from build123d import *

# Parameters (mm, degrees)
SZKIC1_W                                            = 750
SZKIC1_H                                            = 500
WYCI_GNI_CIE1_DEPTH                                 = 80
SFAZOWANIE1_SIZE                                    = 10
WYCI_GNI_CIE2_REACH                                 = 459.739
SZKIC2_R                                            = 52.5
WYCI_GNI_CIE3_REACH                                 = 459.739
SZKIC3_R                                            = 37
SFAZOWANIE2_SIZE                                    = 2
WYTNIJ_WYCI_GNI_CIE1_DEPTH                          = 0.1
SZKIC5_R                                            = 50
WYTNIJ_WYCI_GNI_CIE3_DEPTH                          = 20
POG_BIENIE_WALCOWE_POD_M8_WKR_T_Z_BEM_W_D           = 9
POG_BIENIE_WALCOWE_POD_M8_WKR_T_Z_BEM_W_CBORE_D     = 15
POG_BIENIE_WALCOWE_POD_M8_WKR_T_Z_BEM_W_CBORE_DEPTH = 8.6
OTW_R_POD_RUB_M201_D                                = 22


with BuildPart() as part:
    # Szkic1 → Wyciągnięcie1 (new body)
    with BuildSketch(Plane(origin=(0, 0, 0), x_dir=(1, 0, 0), z_dir=(0, 1, 0))):
        Rectangle(SZKIC1_W, SZKIC1_H)
    extrude(amount=WYCI_GNI_CIE1_DEPTH)

    # Sfazowanie1
    sfazowanie1_edges = [part.edges().sort_by_distance(p)[0] for p in [
        (375, 40, 250),
        (-375, 40, 250),
        (-375, 40, -250),
        (375, 40, -250),
    ]]
    chamfer(sfazowanie1_edges, length=SFAZOWANIE1_SIZE)

    # Szkic2 → Wyciągnięcie2 (cut, up to next)
    with BuildSketch(Plane(origin=(0, 80, 0), x_dir=(1, 0, 0), z_dir=(0, 1, 0)), mode=Mode.PRIVATE) as wyci_gni_cie2_sk1:
        with Locations(Location((-300, 175, 0), (0, 0, 270))):
            Circle(SZKIC2_R)
    wyci_gni_cie2_tool1 = extrude(wyci_gni_cie2_sk1.sketch, amount=-WYCI_GNI_CIE2_REACH, mode=Mode.PRIVATE) & part.part
    # Szkic2 → Wyciągnięcie2 (cut, up to next)
    with BuildSketch(Plane(origin=(0, 80, 0), x_dir=(1, 0, 0), z_dir=(0, 1, 0)), mode=Mode.PRIVATE) as wyci_gni_cie2_sk2:
        with Locations(Location((300, 175, 0), (0, 0, 90))):
            Circle(SZKIC2_R)
    wyci_gni_cie2_tool2 = extrude(wyci_gni_cie2_sk2.sketch, amount=-WYCI_GNI_CIE2_REACH, mode=Mode.PRIVATE) & part.part
    # Szkic2 → Wyciągnięcie2 (cut, up to next)
    with BuildSketch(Plane(origin=(0, 80, 0), x_dir=(1, 0, 0), z_dir=(0, 1, 0)), mode=Mode.PRIVATE) as wyci_gni_cie2_sk3:
        with Locations(Location((-300, -175, 0), (0, 0, 90))):
            Circle(SZKIC2_R)
    wyci_gni_cie2_tool3 = extrude(wyci_gni_cie2_sk3.sketch, amount=-WYCI_GNI_CIE2_REACH, mode=Mode.PRIVATE) & part.part
    # Szkic2 → Wyciągnięcie2 (cut, up to next)
    with BuildSketch(Plane(origin=(0, 80, 0), x_dir=(1, 0, 0), z_dir=(0, 1, 0)), mode=Mode.PRIVATE) as wyci_gni_cie2_sk4:
        with Locations(Location((300, -175, 0), (0, 0, 270))):
            Circle(SZKIC2_R)
    wyci_gni_cie2_tool4 = extrude(wyci_gni_cie2_sk4.sketch, amount=-WYCI_GNI_CIE2_REACH, mode=Mode.PRIVATE) & part.part
    add(wyci_gni_cie2_tool1.solids().sort_by_distance((-300, 80, -175))[0], mode=Mode.SUBTRACT)
    add(wyci_gni_cie2_tool2.solids().sort_by_distance((300, 80, -175))[0], mode=Mode.SUBTRACT)
    add(wyci_gni_cie2_tool3.solids().sort_by_distance((-300, 80, 175))[0], mode=Mode.SUBTRACT)
    add(wyci_gni_cie2_tool4.solids().sort_by_distance((300, 80, 175))[0], mode=Mode.SUBTRACT)

    # Szkic3 → Wyciągnięcie3 (cut, up to next)
    with BuildSketch(Plane(origin=(0, 80, 0), x_dir=(1, 0, 0), z_dir=(0, 1, 0)), mode=Mode.PRIVATE) as wyci_gni_cie3_sk1:
        with Locations(Location((-250, 0, 0), (0, 0, 270))):
            Circle(SZKIC3_R)
    wyci_gni_cie3_tool1 = extrude(wyci_gni_cie3_sk1.sketch, amount=-WYCI_GNI_CIE3_REACH, mode=Mode.PRIVATE) & part.part
    # Szkic3 → Wyciągnięcie3 (cut, up to next)
    with BuildSketch(Plane(origin=(0, 80, 0), x_dir=(1, 0, 0), z_dir=(0, 1, 0)), mode=Mode.PRIVATE) as wyci_gni_cie3_sk2:
        with Locations(Location((250, 0, 0), (0, 0, 90))):
            Circle(SZKIC3_R)
    wyci_gni_cie3_tool2 = extrude(wyci_gni_cie3_sk2.sketch, amount=-WYCI_GNI_CIE3_REACH, mode=Mode.PRIVATE) & part.part
    add(wyci_gni_cie3_tool1.solids().sort_by_distance((-250, 80, 0))[0], mode=Mode.SUBTRACT)
    add(wyci_gni_cie3_tool2.solids().sort_by_distance((250, 80, 0))[0], mode=Mode.SUBTRACT)

    # Sfazowanie2
    sfazowanie2_edges = [part.edges().sort_by_distance(p)[0] for p in [
        (375, 0, 0),
        (375, 80, 0),
        (0, 0, 250),
        (-375, 0, 0),
        (0, 0, -250),
        (-370, 0, 245),
        (-370, 0, -245),
        (370, 0, -245),
        (370, 0, 245),
        (0, 80, 250),
        (0, 80, -250),
        (-375, 80, 0),
        (-370, 80, 245),
        (-370, 80, -245),
        (370, 80, -245),
        (370, 80, 245),
        (-300, 0, -227.5),
        (-300, 80, -227.5),
        (300, 0, -122.5),
        (300, 80, -122.5),
        (-300, 0, 227.5),
        (-300, 80, 227.5),
        (300, 0, 122.5),
        (300, 80, 122.5),
        (-250, 0, -37),
        (-250, 80, -37),
        (250, 0, 37),
        (250, 80, 37),
    ]]
    chamfer(sfazowanie2_edges, length=SFAZOWANIE2_SIZE)

    # Szkic4 → Wytnij-wyciągnięcie1 (cut)
    with BuildSketch(Plane(origin=(0, 0, -250), x_dir=(-1, 0, 0), z_dir=(0, 0, -1))):
        Polygon((-363.299129796, 74.48655724), (-362.394621346, 76.295574139), (-361.625789164, 76.295574139), (-361.625789164, 72.270511538), (-362.394621346, 72.270511538), (-362.394621346, 74.283042838), align=None)
        Polygon((-358.2791079, 76.295574139), (-359.952448532, 73.808175902), (-358.2791079, 73.808175902), (-358.2791079, 72.270511538), (-357.666731233, 72.270511538), (-357.666731233, 76.295574139), align=None)
    extrude(amount=-WYTNIJ_WYCI_GNI_CIE1_DEPTH, mode=Mode.SUBTRACT)

    # Szkic5 → Wytnij-wyciągnięcie3 (cut)
    with BuildSketch(Plane(origin=(0, 80, 0), x_dir=(-1, 0, 0), z_dir=(0, -1, 0))):
        with Locations(Location((0, 0, 0), (0, 0, 90))):
            Circle(SZKIC5_R)
    extrude(amount=WYTNIJ_WYCI_GNI_CIE3_DEPTH, mode=Mode.SUBTRACT)

    # Pogłębienie walcowe pod M8 Wkręt z łbem walcowym z gniazdem sześciokątnym1 (through all)
    with Locations(Plane(origin=(-68.13672833, 0, 0), x_dir=(0, 0, -1), z_dir=(0, -1, 0))):
        with Locations((0, 0), (-59.008137665, 34.068364165), (-59.008137665, 102.205092495), (0, 136.27345666), (59.008137665, 102.205092495), (59.008137665, 34.068364165)):
            CounterBoreHole(POG_BIENIE_WALCOWE_POD_M8_WKR_T_Z_BEM_W_D / 2, POG_BIENIE_WALCOWE_POD_M8_WKR_T_Z_BEM_W_CBORE_D / 2, POG_BIENIE_WALCOWE_POD_M8_WKR_T_Z_BEM_W_CBORE_DEPTH)

    # Otwór pod śrubę M201 (through all)
    with Locations(Plane(origin=(0, 0, 0), x_dir=(-1, 0, 0), z_dir=(0, -1, 0))):
        with Locations((0, 0)):
            Hole(OTW_R_POD_RUB_M201_D / 2)


solid = part.part
Source: CAD feature listing. Evaluate the final solid. Frame: model axes, mm. A direction names the side the tool comes from. Round coordinates to 2 decimals unless told otherwise and drop trailing zeros. Order: outer loops, then holes, each group sorted by start corner. A loop starts at its lowest first (then second) coordinate and runs counter-clockwise, first axis right, second up. Notation, with made-up numbers: (-10.75, 23.25) - (7.25, 23.25) arc R5 cw to (7.25, 29.25) - close; hole circle Ø2 at (61.5, 88). An arc over 180 degrees is marked (long way). Use a Markdown table: item, result. Add a question column.
1. Line query: probe 1 along X at (y, z) = (60, 175); probe 2 along X at (y, z) = (62, 0); probe 3 along Z at (x, y) = (-296, 61.5). Output: solid intervals per line, ascending.
2. Section query C-C (y = 35). Give the number of separate pieces and of enclosed holes in the cut face, then the cut area to 3 significant figures.
3. Section query A-A (x = 300). Return the cut outline in (y, z), then the cut area to 3 significant figures.
4. Section query B-B (x = 0). Return the cut outline in (y, z), then the cut area to 3 significant figures.
5. Set-up query: faces 5 (the cylindrical face through (247.947, 40.532, -168.166)), 6 (the flat face through (12, 60, 1)), 7 (the flat face through (63, 8.6, 0)). Return all of +Z, -Z, +X, -X, +Y, -Y with unobstructed straight access to the full face (end or side cutting, diameter ignored); none if empty.
6. Mould query, pull axis X, two halves, no side actions, for faces 1 (the flat face through (-5, 39, 250)), 2 (the cylindrical face through (-40.722, 4.24, 55.547)), 3 (the flat face through (375, 39, 3)), 4 (the flat face through (-375, 39, 3)). Classes: +X half, -X half, draft (parallel to the pull), parting line (faces both ways), or undercut.
Derived:
| question | item | result |
|---|---|---|
| 1 | probe 1 | -375 to -352.5, -247.5 to 247.5, 352.5 to 375 |
| 1 | probe 2 | -375 to -287, -213 to -72.64, -63.64 to -50, 50 to 63.64, 72.64 to 213, 287 to 375 |
| 1 | probe 3 | -250 to -227.35, -122.65 to 122.65, 227.35 to 250 |
| 2 | separate pieces | 1 |
| 2 | enclosed holes | 13 |
| 2 | area | 331,000 mm2 |
| 3 | outline | (0, -248) - (2, -250) - (78, -250) - (80, -248) - (80, -229.5) - (78, -227.5) - (2, -227.5) - (0, -229.5) - close; (0, -120.5) - (2, -122.5) - (78, -122.5) - (80, -120.5) - (80, 120.5) - (78, 122.5) - (2, 122.5) - (0, 120.5) - close; (0, 229.5) - (2, 227.5) - (78, 227.5) - (80, 229.5) - (80, 248) - (78, 250) - (2, 250) - (0, 248) - close |
| 3 | area | 23,200 mm2 |
| 4 | outline | (0, -248) - (2, -250) - (78, -250) - (80, -248) - (80, -50) - (60, -50) - (60, -11) - (0, -11) - close; (0, 11) - (60, 11) - (60, 50) - (80, 50) - (80, 248) - (78, 250) - (2, 250) - (0, 248) - close |
| 4 | area | 36,700 mm2 |
| 5 | face 5 | +Y, -Y |
| 5 | face 6 | +Y |
| 5 | face 7 | -Y |
| 6 | face 1 | draft |
| 6 | face 2 | undercut |
| 6 | face 3 | +X half |
| 6 | face 4 | -X half |
